Autodesk Inventor part; units mm, degrees
ref_plane "YZ Plane" through (0, 0, 0) normal (1, 0, 0) x (0, 1, 0)
ref_plane "XZ Plane" through (0, 0, 0) normal (0, 1, 0) x (-1, 0, 0)
ref_plane "XY Plane" through (0, 0, 0) normal (0, 0, 1) x (1, 0, 0)
sketch "Náčrt1" plane through (0, 0, 0) normal (0, 1, 0) x (-1, 0, 0)
  line L0 (0, -42) -> (0, 42)
  line L1 (-73.5, 0) -> (73.5, 0)
  line L2 (52.5, 30) -> (-52.5, 30)
  line L3 (-52.5, 30) -> (-52.5, -30)
  line L4 (-52.5, -30) -> (52.5, -30)
  line L5 (52.5, -30) -> (52.5, 30)
  point P0 (0, 0)
  dimension "d0" = 105
  dimension "d1" = 60
extrude "Vysunutí1" add sketch "Náčrt1" along normal blind 50
sketch "Náčrt2" plane through (0, 50, 0) normal (0, 1, 0) x (1, 0, 0)
  line L0 (0, 42) -> (0, -42)
  line L1 (73.5, 0) -> (-73.5, 0)
  point P0 (0, 0)
  point P1 (-48, 25.5)
  point P2 (-48, -25.5)
  point P3 (48, -25.5)
  point P4 (48, 25.5)
  dimension "d4" = 96
  dimension "d5" = 51
  dimension "d6" = 51
  dimension "d7" = 96
  dimension "d8" = 48
  dimension "d9" = 25.5
  dimension "d10" = 25.5
  dimension "d11" = 48
hole "Díra1" at (-48, 50, -25.5) at (-48, 50, 25.5) at (48, 50, 25.5) at (48, 50, -25.5) direction (0, -1, 0) diameter 3.4 end through all
sketch "Náčrt3" plane through (0, 50, 0) normal (0, 1, 0) x (1, 0, 0)
  line L0 (5.5, -13) -> (20.5, -13)
  line L1 (20.5, -13) -> (20.5, -23)
  line L2 (20.5, -23) -> (5.5, -23)
  line L3 (5.5, -23) -> (5.5, -13)
  line L4 (52.5, -30) -> (52.5, 30)
  line L5 (-52.5, -30) -> (52.5, -30)
  point P0 (0, 0)
  dimension "d19" = 15
  dimension "d20" = 10
  dimension "d21" = 32
  dimension "d22" = 7
extrude "Vysunutí2" add sketch "Náčrt3" along normal blind 20
properties part number "prop_PCB"
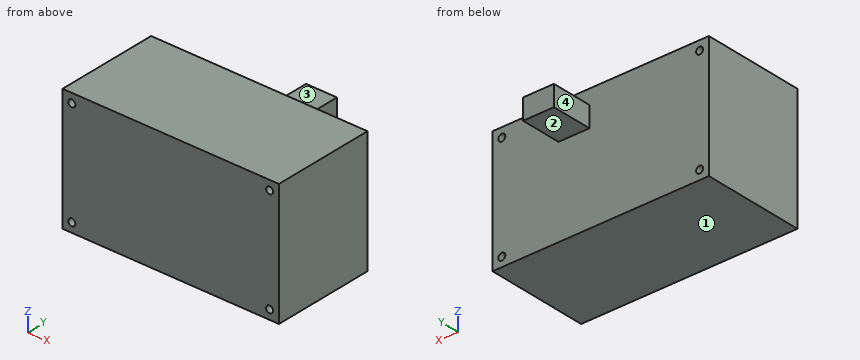
Model file for the job. Use its own axes, mm. Face numbers are marked on the shaded views. A direction names the side the tool comes from. Coordinates: 2 decimals unless noted, no trailing zeros. Loops run counter-clockwise (first coordinate to the right, second up) from the corner with the lowest first, then second, coordinate; pieces in that order, holes last. Notation, with made-up numbers: (-23.75, 73) -> (10.25, 73) arc R17 ccw to (10.25, 84) -> close; hole circle Ø7 at (86, 30). An arc over 180 degrees is marked (long way). Use one line per item in the form item = value. Start each with the question number.
(1) Cut at C-C on z = 14.5. Give the cut face in (x, y).
(2) Cut at B-B on z = 25.5. Give the cut face in (x, y), and give its area (3 significant figures).
(3) Cut at A-A on x = -48. Give the cut face in (y, z).
(4) Tool access for the marked faces 1, 2, 3 and 4: list every direction of +Z, -Z, +X, -X, +Y, -Y with a clear straight run to the whole face (end or side of a thin tool).
(5) Probe probe 1 along Z at (x, y) = (-48, 39); probe 2 along X at (y, z) = (28, 25); probe 3 along X at (y, z) = (36, -24). List the from-to ranges inside material, lowest first. Write a range as from..to.
(6) Flat gauge pins, fed straight in: pin 1 (3 mm diameter, centred on x = -2.5, z = 21, fed in from +Y); pin 2 (3 mm diameter, centred on x = -8, y = 53, fed in from -Z) (3 decimals); pin 3 (16.5 mm diameter, centred on x = 13, y = 62, fed in from -Z); pin 4 (7.5 mm diameter, centred on x = 14.5, y = 62, fed in from +Z). Where does each tip first touch, or does it go through?
(7) Cut at D-D on x = 15. Give the cut face in (y, z), and give its area (3 significant figures).
Values:
q1.outline = (-52.5, 0) -> (52.5, 0) -> (52.5, 50) -> (20.5, 50) -> (20.5, 70) -> (5.5, 70) -> (5.5, 50) -> (-52.5, 50) -> close
q2.outline = (-52.5, 0) -> (-49.7, 0) -> (-49.7, 50) -> (-52.5, 50) -> close; (-46.3, 0) -> (46.3, 0) -> (46.3, 50) -> (-46.3, 50) -> close; (49.7, 0) -> (52.5, 0) -> (52.5, 50) -> (49.7, 50) -> close
q2.area = 4,910 mm2
q3.outline = (0, -30) -> (50, -30) -> (50, -27.2) -> (0, -27.2) -> close; (0, -23.8) -> (50, -23.8) -> (50, 23.8) -> (0, 23.8) -> close; (0, 27.2) -> (50, 27.2) -> (50, 30) -> (0, 30) -> close
q4.face_1 = -Z, +X, -X, +Y, -Y
q4.face_2 = -Z, +X, -X, +Y
q4.face_3 = +Z, +X, -X, +Y
q4.face_4 = +Z, -Z, -X, +Y
q5.probe_1 = -30..-27.2, -23.8..23.8, 27.2..30
q5.probe_2 = -52.5..-49.62, -46.38..46.38, 49.62..52.5
q5.probe_3 = -52.5..-48.8, -47.2..47.2, 48.8..52.5
q6.pin_1 = 50
q6.pin_2 = through
q6.pin_3 = 13
q6.pin_4 = 23
q7.outline = (0, -30) -> (50, -30) -> (50, 13) -> (70, 13) -> (70, 23) -> (50, 23) -> (50, 30) -> (0, 30) -> close
q7.area = 3,200 mm2
